Could you check a few things on this drawing? It's one solid part, dimensions in mm from its lowest x, y, z. A direction names the side the tool comes from. Coordinates: 2 decimals unless noted, no trailing zeros. Write each loop counter-clockwise with the first axis right and the second up, starting at its lowest first coordinate (ties: lowest second). Pieces come first, ordered by that corner, then holes. Notation, with made-up numbers: (54, -39.75) - (82, -39.75) arc R24 cw to (82, -5.75) - close; hole circle Ø6 at (74.5, 77). An arc over 180 degrees is marked (long way). Answer as a JSON object with one key per item and string values. Group by question number.
1) We'd pull the mould along X, two halves only. Please class the marked faces 1, 2 and 3: released by +X, released by -X, zero draft, split by the parting line, or undercut.
2) Will these pins go through, and if not, where does the flat tip stop? pin 1 Ø3 at (y, z) = (6.5, 10) entering from +X; pin 2 Ø1.5 at (y, z) = (12.5, 5.5) entering from -X; pin 3 Ø1.5 at (x, z) = (38, 25.5) entering from +Y; pin 4 Ø1 at (x, y) = (32, 6) entering from -Z.
3) If we section it at D-D (z = 8): Write out the boundary of the cut face in (x, y).
4) On a 3-axis mill with a long thin cutter (end or side, diameter ignored), from which of +Z, -Z, +X, -X, +Y, -Y can I reach the whole of each face in a straight line? I mean the marked faces 4, 5 and 6. Say none if no direction works.
5) If we section it at C-C (x = 24): Write out the boundary of the cut face in (y, z), plus the area to 3 significant figures.
6) Please list where these lines run through material, in increasing order: line 1 along Z through (x, y) = (24, 15.7); line 2 along Z through (x, y) = (43, 1); line 3 along X through (y, z) = (4.25, 14.5).
7) If we section it at B-B (y = 4.5): Write out the boundary of the cut face in (x, z).
8) If we section it at A-A (z = 30): Write out the boundary of the cut face in (x, y).
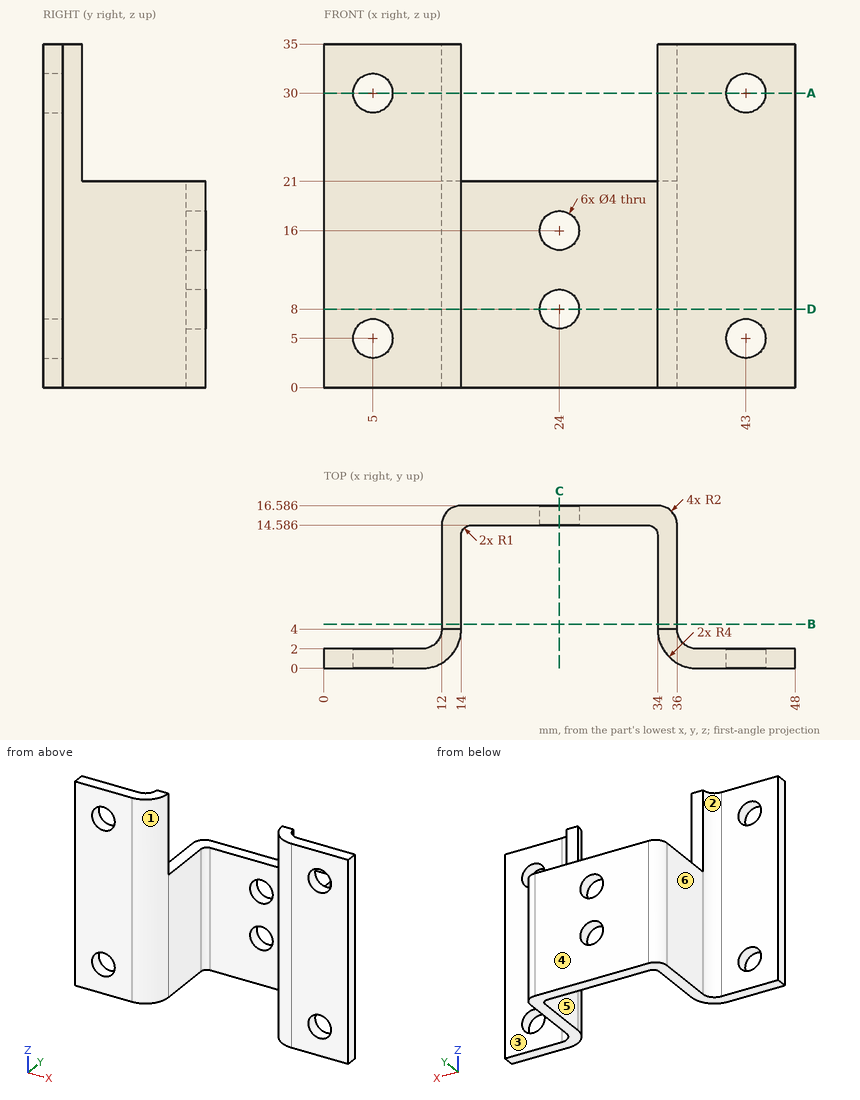
Here are the results:
{
 "1": {"face 1": "undercut", "face 2": "released by -X", "face 3": "zero draft"},
 "2": {"pin 1": "stops at x = 36", "pin 2": "stops at x = 12", "pin 3": "stops at y = 2.15", "pin 4": "passes through"},
 "3": {"outline": "(0, 0) - (10, 0) arc R4 ccw to (14, 4) - (14, 13.59) arc R1 cw to (15, 14.59) - (22, 14.59) - (22, 16.59) - (14, 16.59) arc R2 ccw to (12, 14.59) - (12, 4) arc R2 cw to (10, 2) - (0, 2) - close; (26, 14.59) - (33, 14.59) arc R1 cw to (34, 13.59) - (34, 4) arc R4 ccw to (38, 0) - (48, 0) - (48, 2) - (38, 2) arc R2 cw to (36, 4) - (36, 14.59) arc R2 ccw to (34, 16.59) - (26, 16.59) - close"},
 "4": {"face 4": "+Z, -Z, +X, -X, +Y", "face 5": "+Z, -Z, -Y", "face 6": "+Z, -Z, -X, +Y"},
 "5": {"outline": "(14.59, 0) - (16.59, 0) - (16.59, 6) - (14.59, 6) - close; (14.59, 10) - (16.59, 10) - (16.59, 14) - (14.59, 14) - close; (14.59, 18) - (16.59, 18) - (16.59, 21) - (14.59, 21) - close", "area": "26.0 mm²"},
 "6": {"line 1": "z = 0 to 6, 10 to 14, 18 to 21", "line 2": "z = 0 to 3, 7 to 28, 32 to 35", "line 3": "x = 12 to 14, 34 to 36"},
 "7": {"outline": "(12, 0) - (14, 0) - (14, 21) - (12, 21) - close; (34, 0) - (36, 0) - (36, 21) - (34, 21) - close"},
 "8": {"outline": "(0, 0) - (3, 0) - (3, 2) - (0, 2) - close; (7, 0) - (10, 0) arc R4 ccw to (14, 4) - (12, 4) arc R2 cw to (10, 2) - (7, 2) - close; (34, 4) arc R4 ccw to (38, 0) - (41, 0) - (41, 2) - (38, 2) arc R2 cw to (36, 4) - close; (45, 0) - (48, 0) - (48, 2) - (45, 2) - close"}
}
